Input: part model. Units: mm. Frame: model coordinates. Coordinates: 2 decimals unless noted, no trailing zeros. Loops run counter-clockwise (first coordinate to the right, second up) from the corner with the lowest first, then second, coordinate; pieces in that order, holes last.
```python
from build123d import *

# Parameters (mm, degrees)
BOSS_EXTRUDE1_DEPTH = 4
CUT_EXTRUDE1_REACH  = 9.32
SKETCH4_R           = 2


with BuildPart() as part:
    # Sketch1 → Boss-Extrude1 (new body)
    with BuildSketch(Plane(origin=(0, 0, 0), x_dir=(1, 0, 0), z_dir=(0, 1, 0))):
        Polygon((0, 4.041451884), (-3.5, 2.020725942), (-3.5, -2.020725942), (0, -4.041451884), (3.5, -2.020725942), (3.5, 2.020725942), align=None)
    extrude(amount=BOSS_EXTRUDE1_DEPTH)

    # Sketch2 → Revolve1 (revolve)
    with BuildSketch(Plane.XY, mode=Mode.PRIVATE) as revolve1_sk:
        with BuildLine():
            Line((0, 5), (0, 4))
            Line((0, 4), (3.2, 4))
            Line((3.2, 4), (3.2, 4.4))
            ThreePointArc((3.2, 4.4), (3.024264069, 4.824264069), (2.6, 5))
            Line((2.6, 5), (0, 5))
        make_face()
    revolve(revolve1_sk.sketch.rotate(Axis((0, 0, 0), (0, 1, 0)), 90), axis=Axis((0, 0, 0), (0, 1, 0)))

    # Sketch4 → Cut-Extrude1 (cut, up to next)
    with BuildSketch(Plane.XZ, mode=Mode.PRIVATE) as cut_extrude1_sk1:
        with Locations(Location((0, 0, 0), (0, 0, 270))):
            Circle(SKETCH4_R)
    cut_extrude1_tool1 = extrude(cut_extrude1_sk1.sketch, amount=-CUT_EXTRUDE1_REACH, mode=Mode.PRIVATE) & part.part
    add(cut_extrude1_tool1.solids().sort_by_distance((0, 0, 0))[0], mode=Mode.SUBTRACT)


solid = part.part
```
Item 1: Line query: L1, parallel to X at y = 3.2, z = 0; L2, parallel to Z at x = 2.5, y = 3.7; L3, parallel to Y at x = 3.25, z = 2. Output: solid intervals per line, ascending.
Result:
L1: x = -3.5 to -2, 2 to 3.5
L2: z = -2.6 to 2.6
L3: y = 0 to 4
Item 2: Mould query, pull axis X, two halves, no side actions, for faces 1 (the face through (-2, 0, 2)), 2 (the face through (-0.961, 4.203, -3.052)), 3 (the face through (-2, 2, 0)), 4 (the face through (1.726, 1.972, 3.045)). Classes: +X half, -X half, draft (parallel to the pull), parting line (faces both ways), or undercut.
Result:
face 1: draft
face 2: parting line
face 3: undercut
face 4: +X half
Item 3: Section query B-B (y = 3.55). Output: boundary loops of the cut face in (x, z).
Result:
outline: (-3.5, -2.02) - (0, -4.04) - (3.5, -2.02) - (3.5, 2.02) - (0, 4.04) - (-3.5, 2.02) - close; hole circle Ø4 at (0, 0)
Item 4: Section query A-A (z = 0). Output: boundary loops of the cut face in (x, y), then the cut area to 3 significant figures.
Result:
outline: (-3.5, 0) - (-2, 0) - (-2, 5) - (-2.6, 5) arc R0.6 ccw to (-3.2, 4.4) - (-3.2, 4) - (-3.5, 4) - close; (2, 0) - (3.5, 0) - (3.5, 4) - (3.2, 4) - (3.2, 4.4) arc R0.6 ccw to (2.6, 5) - (2, 5) - close
area: 14.2 mm2
Item 5: Contact query for a flat-ended pin moving along its axis: P1, Ø3, axis at x = -2, y = 4.5, coming from the -Z side. Output: stop coordinate, or through.
Result:
P1: stops at z = -3.7
Item 6: Section query C-C (z = -3.5). Output: boundary loops of the cut face in (x, y).
Result:
outline: (-0.94, 0) - (0.94, 0) - (0.94, 4) - (-0.94, 4) - close
